Geometry check sheet. Reference: the model listing, model coordinates, mm. Face numbers are marked on the shaded views. Give positions to 0.01 mm unless a question says otherwise; leave off trailing zeros. Order: outer loops, then holes, each group sorted by start corner. A loop starts at its lowest first (then second) coordinate and runs counter-clockwise, first axis right, second up. Notation, with made-up numbers: M -40,63 L -4,63 A12 cw -4,81 Z; hole C 21.5,-18.75 d9. An arc over 180 degrees is marked long. Use CSV: the item, a comma, the result in double quotes. Start each with the question number.
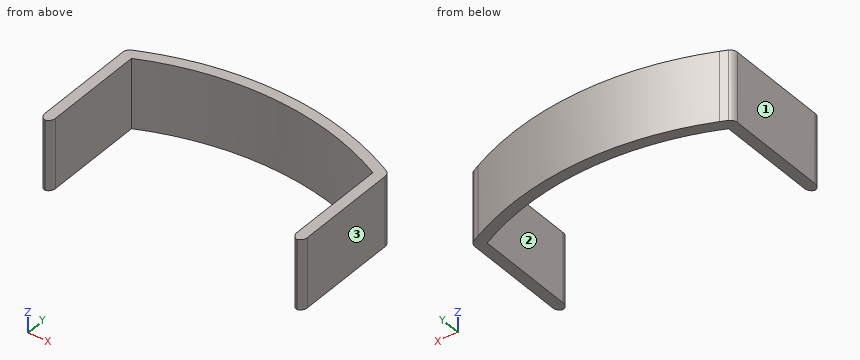
from build123d import *

# Parameters (mm, degrees)
F1_DEPTH    = 12.7
F3_DEPTH    = 32.1945
F4_T1_DEPTH = 19.05
F5_R        = 1.27


# Not quite as in the source:
# - a fillet or chamfer that OpenCascade refuses, or shapes differently, is made with other operations: its cross-section is extruded or revolved along the edge and cut away or added


with BuildPart() as f1:
    # F0 (on Top) → F1 (new body)
    with BuildSketch(Plane.XY):
        with BuildLine():
            Line((-25.9680064888, 45.8637074821), (-25.9680064888, 43.6612258073))
            ThreePointArc((-25.9680064888, 43.6612258073), (-23.9313543809, 44.8099350312), (-21.844, 45.8637074821))
            Line((-21.844, 45.8637074821), (-21.844, 47.9651612006))
            ThreePointArc((-21.844, 47.9651612006), (-23.929083101, 46.9597275008), (-25.9680064888, 45.8637074821))
        make_face()
        with BuildLine():
            ThreePointArc((-21.844, 45.8637074821), (-23.9313543809, 44.8099350312), (-25.9680064888, 43.6612258073))
            Line((-25.9680064888, 43.6612258073), (-25.9680064888, 26.8137074821))
            Line((-25.9680064888, 26.8137074821), (-21.844, 26.8137074821))
            Line((-21.844, 26.8137074821), (-21.844, 45.8637074821))
        make_face()
        with BuildLine():
            ThreePointArc((21.844, 45.8637074821), (23.9313543809, 44.8099350312), (25.9680064888, 43.6612258073))
            Line((25.9680064888, 43.6612258073), (25.9680064888, 45.8637074821))
            ThreePointArc((25.9680064888, 45.8637074821), (23.929083101, 46.9597275008), (21.844, 47.9651612006))
            Line((21.844, 47.9651612006), (21.844, 45.8637074821))
        make_face()
        with BuildLine():
            Line((25.9680064888, 26.8137074821), (25.9680064888, 43.6612258073))
            ThreePointArc((25.9680064888, 43.6612258073), (23.9313543809, 44.8099350312), (21.844, 45.8637074821))
            Line((21.844, 45.8637074821), (21.844, 26.8137074821))
            Line((21.844, 26.8137074821), (25.9680064888, 26.8137074821))
        make_face()
        with BuildLine():
            ThreePointArc((-21.844, 45.8637074821), (0, 50.8), (21.844, 45.8637074821))
            Line((21.844, 45.8637074821), (21.844, 47.9651612006))
            ThreePointArc((21.844, 47.9651612006), (0, 52.705), (-21.844, 47.9651612006))
            Line((-21.844, 47.9651612006), (-21.844, 45.8637074821))
        make_face()
    extrude(amount=F1_DEPTH)

    # F2 (on face) → F3 (cut, symmetric)
    with BuildSketch(Plane.XY.offset(12.7)):
        with BuildLine():
            Line((-23.749, 47.0510576289), (-23.749, 52.2757731378))
            Line((-23.749, 52.2757731378), (-31.0743017153, 52.1406124749))
            Line((-31.0743017153, 52.1406124749), (-30.5507772572, 23.7671602517))
            Line((-30.5507772572, 23.7671602517), (-23.749, 23.7671602517))
            Line((-23.749, 23.7671602517), (-23.749, 26.8137074821))
            Line((-23.749, 26.8137074821), (-25.9680064888, 26.8137074821))
            Line((-25.9680064888, 26.8137074821), (-25.9680064888, 45.8637074821))
            ThreePointArc((-25.9680064888, 45.8637074821), (-24.8655913592, 46.4706293411), (-23.749, 47.0510576289))
        make_face()
        with BuildLine():
            Line((23.749, 52.2757731378), (23.749, 47.0510576289))
            ThreePointArc((23.749, 47.0510576289), (24.8655913592, 46.4706293411), (25.9680064888, 45.8637074821))
            Line((25.9680064888, 45.8637074821), (25.9680064888, 26.8137074821))
            Line((25.9680064888, 26.8137074821), (23.749, 26.8137074821))
            Line((23.749, 26.8137074821), (23.749, 23.7671602517))
            Line((23.749, 23.7671602517), (30.5507772572, 23.7671602517))
            Line((30.5507772572, 23.7671602517), (31.0743017153, 52.1406124749))
            Line((31.0743017153, 52.1406124749), (23.749, 52.2757731378))
        make_face()
        with BuildLine():
            Line((-23.749, 26.8137074821), (-23.749, 47.0510576289))
            ThreePointArc((-23.749, 47.0510576289), (-24.8655913592, 46.4706293411), (-25.9680064888, 45.8637074821))
            Line((-25.9680064888, 45.8637074821), (-25.9680064888, 26.8137074821))
            Line((-25.9680064888, 26.8137074821), (-23.749, 26.8137074821))
        make_face()
        with BuildLine():
            ThreePointArc((25.9680064888, 45.8637074821), (24.8655913592, 46.4706293411), (23.749, 47.0510576289))
            Line((23.749, 47.0510576289), (23.749, 26.8137074821))
            Line((23.749, 26.8137074821), (25.9680064888, 26.8137074821))
            Line((25.9680064888, 26.8137074821), (25.9680064888, 45.8637074821))
        make_face()
    extrude(amount=F3_DEPTH, both=True, mode=Mode.SUBTRACT)

    # F4: fillet of radius 1.27 on 4 edges, made by hand

    # F4_s2 → F4_t1 (cut)
    with BuildSketch(Plane.XY.offset(-3.175)):
        with BuildLine():
            ThreePointArc((-21.844, 28.0837074821), (-22.2159743879, 27.18568187), (-23.114, 26.8137074821))
            Line((-23.114, 26.8137074821), (-21.844, 26.8137074821))
            Line((-21.844, 26.8137074821), (-21.844, 28.0837074821))
        make_face()
        with BuildLine():
            ThreePointArc((-23.749, 28.0837074821), (-23.3770256121, 27.18568187), (-22.479, 26.8137074821))
            Line((-22.479, 26.8137074821), (-23.749, 26.8137074821))
            Line((-23.749, 26.8137074821), (-23.749, 28.0837074821))
        make_face()
        with BuildLine():
            ThreePointArc((23.114, 26.8137074821), (22.2159743879, 27.18568187), (21.844, 28.0837074821))
            Line((21.844, 28.0837074821), (21.844, 26.8137074821))
            Line((21.844, 26.8137074821), (23.114, 26.8137074821))
        make_face()
        with BuildLine():
            ThreePointArc((23.749, 28.0837074821), (23.3770256121, 27.18568187), (22.479, 26.8137074821))
            Line((22.479, 26.8137074821), (23.749, 26.8137074821))
            Line((23.749, 26.8137074821), (23.749, 28.0837074821))
        make_face()
    extrude(amount=F4_T1_DEPTH, mode=Mode.SUBTRACT)

    # F5
    f5_edges = [f1.edges().sort_by_distance(p)[0] for p in [
        (23.749, 47.051058, 6.35),
        (-23.749, 47.051058, 6.35),
    ]]
    fillet(f5_edges, radius=F5_R)


solid = f1.part
(1) Sectioned sample at B-B on z = 8. Record the cut outline in (x, y) (1 decimal), then the cut area to 3 significant figures.
(2) Go/stop test with flat-tipped pins: P1, Ø4, axis at x = -12.5, z = 6, coming from the +Y side; P2, Ø2, axis at x = 2.5, z = 3, coming from the -Y side; P3, Ø3, axis at x = 9.5, z = 9.5, coming from the -Y side. Record where each tip stops, or that it passes through.
(3) Sectioned sample at C-C on x = -0.5. Record the cut outline in (y, z).
(4) Draft check along X on the marked faces 1, 2 and 3. Enter one of: +X half, -X half, draft (parallel to the pull), parting line (faces both ways), or undercut.
(5) Sectioned sample at A-A on y = 34.5. Record the cut outline in (x, z), then the cut area to 3 significant figures.
(6) Sectioned sample at D-D on y = 50.25. Record the cut outline in (x, z), then the cut area to 3 significant figures.
(7) Thickness scan on line 1 (X direction, y = 28.75, z = 3.25); line 2 (X direction, y = 46.75, z = 2.75); line 3 (Y direction, x = 0.5, z = 10.25). Record the ranges inside material, lowest first.
Responses:
1,outline,"M -23.7,28.1 A1.3 ccw -22.8,26.9 A1.3 ccw -21.8,28.1 L -21.8,45.9 A50.8 cw 21.8,45.9 L 21.8,28.1 A1.3 ccw 22.8,26.9 A1.3 ccw 23.7,28.1 L 23.7,46.3 A1.3 ccw 23,47.4 A52.7 ccw -23,47.4 A1.3 ccw -23.7,46.3 Z"
1,area,"163 mm2"
2,P1,"y = 51.65"
2,P2,"y = 50.68"
2,P3,"y = 49.59"
3,outline,"M 50.8,0 L 52.7,0 L 52.7,12.7 L 50.8,12.7 Z"
4,face 1,"-X half"
4,face 2,"undercut"
4,face 3,"+X half"
5,outline,"M -23.75,0 L -21.84,0 L -21.84,12.7 L -23.75,12.7 Z; M 21.84,0 L 23.75,0 L 23.75,12.7 L 21.84,12.7 Z"
5,area,"48.4 mm2"
6,outline,"M -15.9,0 L -7.46,0 L -7.46,12.7 L -15.9,12.7 Z; M 7.46,0 L 15.9,0 L 15.9,12.7 L 7.46,12.7 Z"
6,area,"214 mm2"
7,line 1,"-23.75 to -21.84, 21.84 to 23.75"
7,line 2,"-23.65 to -19.88, 19.88 to 23.65"
7,line 3,"50.8 to 52.7"
